Source: CAD feature listing. Evaluate the final solid. Frame: model axes, mm. A direction names the side the tool comes from. Round coordinates to 2 decimals unless told otherwise and drop trailing zeros. Order: outer loops, then holes, each group sorted by start corner. A loop starts at its lowest first (then second) coordinate and runs counter-clockwise, first axis right, second up. Notation, with made-up numbers: (-22.5, -6) -> (-13.5, -6) arc R13 cw to (-13.5, 9) -> close; hole circle Ø11 at (12, 44). An arc over 180 degrees is marked (long way). One line per item, written item: value. Start each with the question number.
1) Ray query, L1, parallel to Z at x = -0.5, y = 3.75; L2, parallel to Z at x = 3.75, y = -6.5; L3, parallel to Y at x = -0.5, z = 3. Return the intervals inside material, ascending.
2) Section A-A (x = 0). Return the cut outline in (y, z).
3) Section D-D (z = 5.5). Return the cut outline in (x, y).
4) Pin query (flat end, axial travel): P1, Ø5.5, axis at x = 1, y = 2, coming from the -Z side; P2, Ø4, axis at x = 0.5, z = 2.5, coming from the -Y side; P3, Ø1.5, axis at y = 2.5, z = 1, coming from the -X side; P4, Ø6.5, axis at x = 4.5, y = -0.5, coming from the -Z side. Return the tip coordinate at first contact, or that it passes through.
5) Reachability of faces 1 (the face through (-0.1, -2.4, 5)), 2 (the face through (0, 0, 0)) from +Z, -Z, +X, -X, +Y, -Y: full face, straight path, thin tool, end or side. Return the list, or none.
6) Section C-C (z = 2). Return the cut outline in (x, y), and give its area (3 significant figures).
```python
from build123d import *

# Parameters (mm, degrees)
F0_R     = 1.95
F1_DEPTH = 5
F2_R     = 5.5
F2_R_2   = 1.95
F3_DEPTH = 1
F4_R     = 11
F5_DEPTH = 1.5
F6_SIZE  = 1


with BuildPart() as f1:
    # F0 (on Top) → F1 (new body)
    with BuildSketch(Plane.XY):
        Circle(F0_R)
    extrude(amount=F1_DEPTH)

    # F2 (on face) → F3 (join)
    with BuildSketch(Plane.XY.offset(5)):
        Circle(F2_R)
        Circle(F2_R_2, mode=Mode.SUBTRACT)
        Circle(F2_R_2)
    extrude(amount=F3_DEPTH)

    # F4 (on face) → F5 (join)
    with BuildSketch(Plane.XY.offset(6)):
        Circle(F4_R)
    extrude(amount=F5_DEPTH)

    # F6
    f6_edges = [f1.edges().sort_by_distance(p)[0] for p in [
        (-11, 0, 7.5),
        (-1.95, 0, 0),
    ]]
    chamfer(f6_edges, length=F6_SIZE)


solid = f1.part
```
Findings:
1. L1: 5 to 7.5
1. L2: 6 to 7.5
1. L3: -1.88 to 1.88
2. outline: (-11, 6) -> (-5.5, 6) -> (-5.5, 5) -> (-1.95, 5) -> (-1.95, 1) -> (-0.95, 0) -> (0.95, 0) -> (1.95, 1) -> (1.95, 5) -> (5.5, 5) -> (5.5, 6) -> (11, 6) -> (11, 6.5) -> (10, 7.5) -> (-10, 7.5) -> (-11, 6.5) -> close
3. outline: circle Ø11 at (0, 0)
4. P1: z = 0
4. P2: y = -1.95
4. P3: x = -0.86
4. P4: z = 0.33
5. face 1: -Z
5. face 2: -Z, +X, -X, +Y, -Y
6. outline: circle Ø3.9 at (0, 0)
6. area: 11.9 mm2
